Geometry check sheet. Reference: the model listing, model coordinates, mm. Coordinates: 2 decimals unless noted, no trailing zeros. Write each loop counter-clockwise with the first axis right and the second up, starting at its lowest first coordinate (ties: lowest second). Pieces come first, ordered by that corner, then holes. Notation, with made-up numbers: M 51.25,39.5 L 60.25,39.5 A16 ccw 60.25,66.5 Z; hole C 6,60.5 d6. An arc over 180 degrees is marked long. Put each result on its own line as item: value. Start each with the question number.
1) Gauge pin test, flat ends, axial feed: pin 1 (1 mm diameter, centred on y = 2, z = 13, fed in from +X); pin 2 (1.5 mm diameter, centred on x = 15, y = 0.5, fed in from +Z); pin 3 (5.5 mm diameter, centred on x = 0, z = 0, fed in from -Y); pin 4 (1.5 mm diameter, centred on y = 2, z = -14.5, fed in from -X). Record the tip position at first contact, or that the pin passes through.
2) Cross-section at B-B on y = 1.8. Record the cut outline in (x, z).
3) Cross-section at A-A on x = 0. Record the cut outline in (y, z) (3 decimals), plus the area to 3 significant figures.
4) Mould release check, pull along X, two halves, no side actions. Record for faces 1 (the cylindrical face through (26.686, 1.394, -0.221)), 2 (the flat face through (-6, 3, 0)), 3 (the cylindrical face through (-24.397, 1.417, 12.69)): released by +X, released by -X, zero draft, split by the parting line, or undercut.
5) Cross-section at C-C on z = 0. Record the cut outline in (x, y) (3 decimals), plus the area to 3 significant figures.
6) Scan lines: line 1 along X through (y, z) = (0.85, 0); line 2 along X through (y, z) = (2.4, -1); line 3 along X through (y, z) = (1, 25). Record each from-to range of solid material in increasing order.
from build123d import *

# Parameters (mm, degrees)
SKETCH1_R           = 27.5
SKETCH1_R_2         = 3.3
BOSS_EXTRUDE1_DEPTH = 3
SKETCH2_R           = 1.7
CUT_EXTRUDE1_DEPTH  = 40.00640973
CHAMFER1_SIZE       = 0.125
FILLET1_R           = 0.25


with BuildPart() as part:
    # Sketch1 → Boss-Extrude1 (new body)
    with BuildSketch(Plane(origin=(0, 0, 0), x_dir=(1, 0, 0), z_dir=(0, 1, 0))):
        with Locations(Location((0, 0, 0), (0, 0, 270))):
            Circle(SKETCH1_R)
        with Locations(Location((0, 0, 0), (0, 0, 270))):
            Circle(SKETCH1_R_2, mode=Mode.SUBTRACT)
    extrude(amount=BOSS_EXTRUDE1_DEPTH)

    # Sketch2 → Cut-Extrude1 (cut, through all)
    with BuildSketch(Plane(origin=(0, 3, 0), x_dir=(1, 0, 0), z_dir=(0, 1, 0))):
        with Locations(Location((-25, 0, 0), (0, 0, 270))):
            Circle(SKETCH2_R)
        with Locations(Location((0, -25, 0), (0, 0, 270))):
            Circle(SKETCH2_R)
        with Locations(Location((25, 0, 0), (0, 0, 270))):
            Circle(SKETCH2_R)
        with Locations(Location((0, 25, 0), (0, 0, 270))):
            Circle(SKETCH2_R)
    extrude(amount=-CUT_EXTRUDE1_DEPTH, mode=Mode.SUBTRACT)

    # Chamfer1
    chamfer1_edges = [part.edges().sort_by_distance(p)[0] for p in [
        (0, 3, -27.5),
    ]]
    chamfer(chamfer1_edges, length=CHAMFER1_SIZE)

    # Fillet1
    fillet1_edges = [part.edges().sort_by_distance(p)[0] for p in [
        (-25, 3, -1.7),
        (0, 3, 23.3),
        (25, 3, -1.7),
        (0, 3, -26.7),
    ]]
    fillet(fillet1_edges, radius=FILLET1_R)


solid = part.part
Answer key:
1. pin 1: stops at x = 24.49
1. pin 2: stops at z = 23.52
1. pin 3: passes through
1. pin 4: stops at x = -23.82
2. outline: C 0,0 d55; hole C -25,0 d3.4; hole C 0,0 d6.6; hole C 0,-25 d3.4; hole C 0,25 d3.4; hole C 25,0 d3.4
3. outline: M 0,-27.5 L 2.875,-27.5 L 3,-27.375 L 3,-26.95 A0.25 ccw 2.75,-26.7 L 0,-26.7 Z; M 0,-23.3 L 2.75,-23.3 A0.25 ccw 3,-23.05 L 3,-3.3 L 0,-3.3 Z; M 0,3.3 L 3,3.3 L 3,23.05 A0.25 ccw 2.75,23.3 L 0,23.3 Z; M 0,26.7 L 2.75,26.7 A0.25 ccw 3,26.95 L 3,27.375 L 2.875,27.5 L 0,27.5 Z
3. area: 125 mm²
4. face 1: undercut
4. face 2: zero draft
4. face 3: split by the parting line
5. outline: M -27.5,0 L -26.7,0 L -26.7,2.75 A0.25 ccw -26.95,3 L -27.375,3 L -27.5,2.875 Z; M -23.3,0 L -3.3,0 L -3.3,3 L -23.05,3 A0.25 ccw -23.3,2.75 Z; M 3.3,0 L 23.3,0 L 23.3,2.75 A0.25 ccw 23.05,3 L 3.3,3 Z; M 26.7,0 L 27.5,0 L 27.5,2.875 L 27.375,3 L 26.95,3 A0.25 ccw 26.7,2.75 Z
5. area: 125 mm²
6. line 1: x = -27.5 to -26.7, -23.3 to -3.3, 3.3 to 23.3, 26.7 to 27.5
6. line 2: x = -27.48 to -26.37, -23.63 to -3.14, 3.14 to 23.63, 26.37 to 27.48
6. line 3: x = -11.46 to -1.7, 1.7 to 11.46
